Could you check a few things on this model? Use its own coordinates, in mm. Face numbers are marked on the shaded views. A direction names the side the tool comes from. Coordinates: 2 decimals unless noted, no trailing zeros. Write each loop counter-clockwise with the first axis right and the second up, starting at its lowest first coordinate (ties: lowest second). Pieces come first, ordered by that corner, then holes. Notation, with made-up numbers: (23, -9.5) - (59, -9.5) arc R30 ccw to (59, 20.5) - close; hole circle Ø8 at (-12, 66.5). An arc over 180 degrees is marked (long way). Answer as a JSON object with one key per item and string values. Group by question number.
1) If we section it at C-C (y = -92): Write out the boundary of the cut face in (x, z).
2) Will these pins go through, and if not, where does the flat tip stop? pin 1 Ø3 at (x, z) = (0, 35.5) entering from -Y; pin 2 Ø6 at (x, z) = (-10.5, 29.5) entering from -Y; pin 3 Ø6 at (y, z) = (-52.5, 56) entering from +X; pin 4 Ø6 at (x, z) = (5, 80.5) entering from +Y.
3) If we section it at B-B (x = -22): Write out the boundary of the cut face in (y, z).
4) If we section it at A-A (y = -50.8): Write out the boundary of the cut face in (x, z), plus the area to 3 significant figures.
5) Please list where these lines run through material, in increasing order: line 1 along Z through (x, y) = (1, -35); line 2 along Y through (x, z) = (-4, 54); line 3 along Y through (x, z) = (4.5, 112.5).
6) On a 3-axis mill with a long thin cutter (end or side, diameter ignored), from which of +Z, -Z, +X, -X, +Y, -Y can I reach the whole of each face in a straight line? I mean the marked faces 1 and 2. Say none if no direction works.
```python
from build123d import *

# Parameters (mm, degrees)
F1_DEPTH = 101.6
F2_R     = 15.24
F3_DEPTH = 101.6
F4_SIZE  = 2.54


with BuildPart() as f1:
    # F0 (on Front) → F1 (new body)
    with BuildSketch(Plane.XZ):
        Polygon((27.494166, 29.467992), (0, 29.467992), (-33.607345, 29.467992), (-33.607345, -21.700272), (27.494166, -21.700272), align=None)
    extrude(amount=F1_DEPTH)

    # F2 (on face) → F3 (join)
    with BuildSketch(Plane.XY.offset(29.467992)):
        with Locations((-3.05659, -50.8)):
            Circle(F2_R)
    extrude(amount=F3_DEPTH)

    # F4
    f4_edges = [f1.edges().sort_by_distance(p)[0] for p in [
        (-18.29659, -50.8, 131.067992),
    ]]
    chamfer(f4_edges, length=F4_SIZE)


solid = f1.part
```
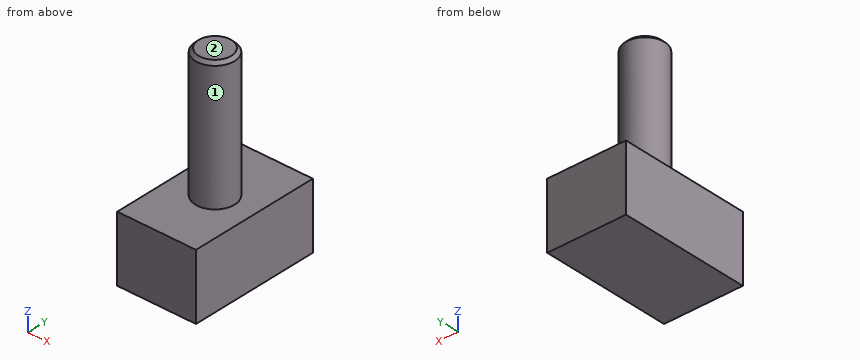
Here are the results:
{
 "1": {"outline": "(-33.61, -21.7) - (27.49, -21.7) - (27.49, 29.47) - (-33.61, 29.47) - close"},
 "2": {"pin 1": "stops at y = -65.96", "pin 2": "stops at y = -101.6", "pin 3": "stops at x = 12.18", "pin 4": "stops at y = -36.42"},
 "3": {"outline": "(-101.6, -21.7) - (0, -21.7) - (0, 29.47) - (-101.6, 29.47) - close"},
 "4": {"outline": "(-33.61, -21.7) - (27.49, -21.7) - (27.49, 29.47) - (12.18, 29.47) - (12.18, 128.53) - (9.64, 131.07) - (-15.76, 131.07) - (-18.3, 128.53) - (-18.3, 29.47) - (-33.61, 29.47) - close", "area": "6,220 mm²"},
 "5": {"line 1": "z = -21.7 to 29.47", "line 2": "y = -66.01 to -35.59", "line 3": "y = -64.03 to -37.57"},
 "6": {"face 1": "+Z", "face 2": "+Z, +X, -X, +Y, -Y"}
}
